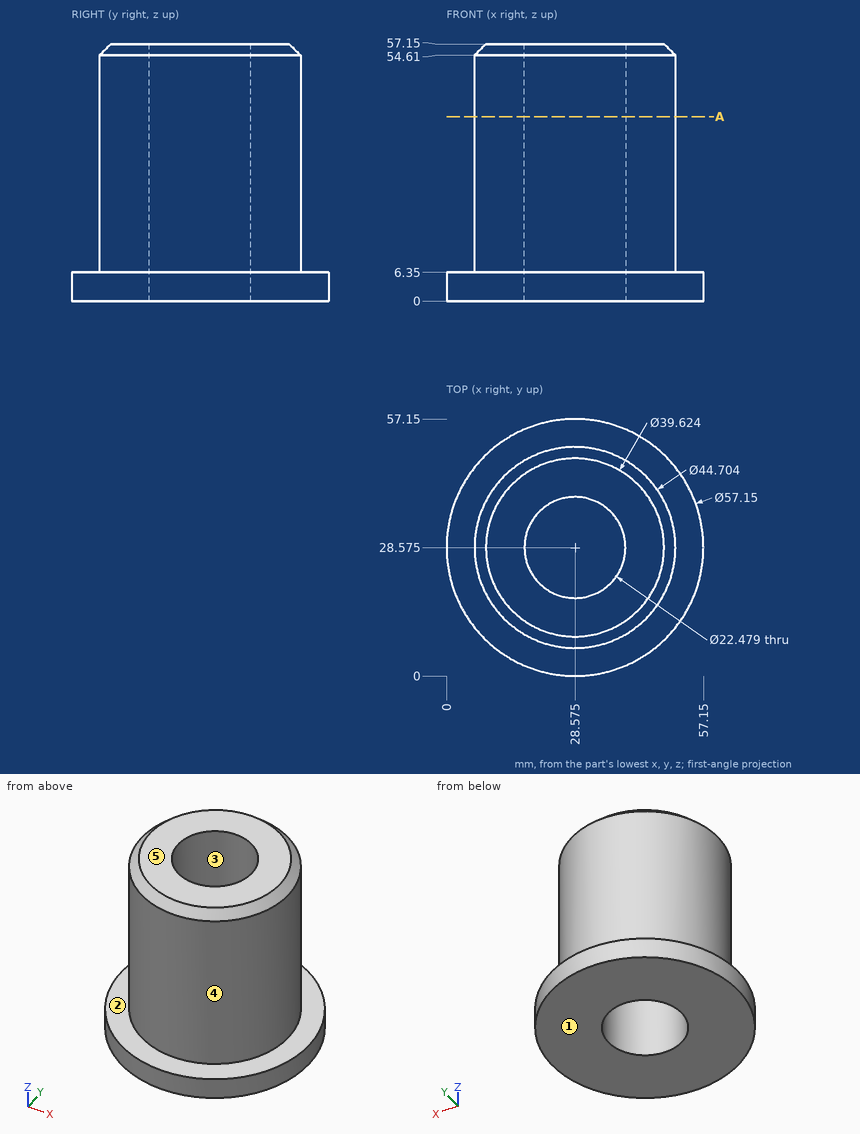
Could you check a few things on this drawing? It's one solid part, dimensions in mm from its lowest x, y, z. A direction names the side the tool comes from. Round coordinates to 2 decimals unless told otherwise and drop trailing zeros. Loops run counter-clockwise (first coordinate to the right, second up) from the corner with the lowest first, then second, coordinate; pieces in that order, holes last. Notation, with made-up numbers: (39, 7.5) -> (54, 7.5) arc R23 cw to (54, 39.5) -> close; hole circle Ø8 at (10, 76). An arc over 180 degrees is marked (long way). One line per item, written item: value. Start each with the question number.
1. If we section it at A-A, the plane z = 41: Write out the boundary of the cut face in (x, y) (1 decimal).
2. If we mould it in two halves opening along Y, with no side actions, what happens to the marked faces 3, 4 and 5? For each: pulls with the +Y half, pulls with the -Y half, needs draft (parallel to the pull), parting line crosses it, or undercut.
3. For the marked faces 1 and 2, which set-ups out of +Z, -Z, +X, -X, +Y, -Y let a thin tool reach every point of the face, with its end or its side?
4. For pin 1 (5 mm diameter, centred on y = 47.5, z = 48, fed in from +X); pin 2 (12 mm diameter, centred on x = 9, y = 9.5, fed in from +Z); pin 3 (2 mm diameter, centred on x = 31.5, z = 43, fed in from -Y), each with a flat end and sliding along its axis, tell me the tip position at first contact or that it passes through.
5. If I drill on probe 1 along Z at (x, y) = (7.5, 39.5); probe 2 along Y at (x, z) = (25, 8.5); probe 3 along Y at (x, z) = (38, 15.5), over which ranges is the centre line in solid material (lowest first)?
Calculated:
1. outline: circle Ø44.7 at (28.6, 28.6); hole circle Ø22.5 at (28.6, 28.6)
2. face 3: undercut
2. face 4: parting line crosses it
2. face 5: needs draft
3. face 1: -Z, +X, -X, +Y, -Y
3. face 2: +Z
4. pin 1: stops at x = 43.74
4. pin 2: stops at z = 55.63
4. pin 3: stops at y = 6.31
5. probe 1: z = 0 to 6.35
5. probe 2: y = 6.51 to 17.92, 39.23 to 50.64
5. probe 3: y = 8.31 to 22.45, 34.7 to 48.84
